Autodesk Inventor part; units mm, degrees
ref_plane "YZ Plane" through (0, 0, 0) normal (1, 0, 0) x (0, 1, 0)
ref_plane "XZ Plane" through (0, 0, 0) normal (0, 1, 0) x (-1, 0, 0)
ref_plane "XY Plane" through (0, 0, 0) normal (0, 0, 1) x (1, 0, 0)
sketch "Sketch1" plane through (0, 0, 0) normal (0, 0, 1) x (1, 0, 0)
  line L0 (0, 0) -> (310, 0)
  line L1 (310, 0) -> (310, 40)
  line L2 (310, 40) -> (0, 40)
  line L3 (0, 40) -> (0, 0)
  dimension "d1" = 40
  dimension "d2" = 310
extrude "Plate1" add sketch "Sketch1" along normal blind 2
sketch "Sketch2" plane through (310, 38, 2) normal (0, 1, 0) x (-1, 0, 0)
  line L0 (310, 0) -> (0, 0)
  line L1 (0, 0) -> (0, -25)
  line L2 (0, -25) -> (310, -25)
  line L3 (310, -25) -> (310, 0)
edge flange "Flange1" height 25 angle 90 thickness 2 bend radius 2 thickness toward (0, 1, 0) relief tear relief width 2 relief depth 1 edges at (155, 40, 0) wall of the first edge with corners at (0, 38, 2) (310, 38, 2) (310, 38, -23) (0, 38, -23)
bend "Bend1"
corner "Corner1"
sketch "Sketch3" plane through (0, 2, 2) normal (0, -1, 0) x (1, 0, 0)
  line L0 (310, 0) -> (0, 0)
  line L1 (0, 0) -> (0, -12)
  line L2 (0, -12) -> (310, -12)
  line L3 (310, -12) -> (310, 0)
edge flange "Flange2" height 12 angle 90 thickness 2 bend radius 2 thickness toward (0, -1, 0) relief tear relief width 2 relief depth 1 edges at (155, 0, 0) wall of the first edge with corners at (310, 2, 2) (0, 2, 2) (0, 2, -10) (310, 2, -10)
bend "Bend2"
corner "Corner2"
sketch "Sketch4" plane through (0, 0, 2) normal (0, 0, 1) x (1, 0, 0)
  arc A0 (146.75, 13.9172) -> (163.25, 13.9172) centre (155, 20) ccw
  line L0 (0, 4) -> (0, 36)
  line L1 (0, 40) -> (310, 40)
  line L2 (146.75, 26.0828) -> (146.75, 13.9172)
  line L3 (163.25, 26.0828) -> (163.25, 13.9172)
  arc A1 (146.75, 26.0828) -> (146.75, 13.9172) centre (155, 20) ccw construction
  arc A2 (163.25, 26.0828) -> (146.75, 26.0828) centre (155, 20) ccw
  arc A3 (163.25, 13.9172) -> (163.25, 26.0828) centre (155, 20) ccw construction
  point P0 (0, 0)
  point P1 (0, 20)
  point P2 (155, 40)
  dimension "d25" = 20.5
  dimension "d26" = 16.5
extrude "Cut1" cut sketch "Sketch4" against normal blind 2
sketch "Sketch5" plane through (0, 0, 2) normal (0, 0, 1) x (1, 0, 0)
  line L0 (310, 4) -> (0, 4)
  line L1 (145, 4) -> (165, 4)
  line L2 (165, 4) -> (165, -2)
  line L3 (165, -2) -> (145, -2)
  line L4 (145, -2) -> (145, 4)
  point P0 (0, 0)
  point P1 (155, -2)
  point P2 (155, 4)
  dimension "d27" = 20
  dimension "d28" = 6
extrude "Cut2" cut sketch "Sketch5" against normal through all
equation "\"d23\" = Thickness"
equation "\"d29\" = Thickness"
equation "\"d3\" = BendReliefWidth"
equation "\"d4\" = BendReliefDepth"
equation "\"d5\" = MinimumRemnant"
equation "\"d6\" = BendRadius"
equation "\"d9\" = BendRadius"
equation "\"d10\" = CornerReliefSize"
equation "\"d11\" = GapSize"
equation "\"d12\" = JacobiRadiusSize"
equation "\"d13\" = BendReliefWidth"
equation "\"d14\" = BendReliefDepth"
equation "\"d15\" = MinimumRemnant"
equation "\"d16\" = BendRadius"
equation "\"d19\" = BendRadius"
equation "\"d20\" = CornerReliefSize"
equation "\"d21\" = GapSize"
equation "\"d22\" = JacobiRadiusSize"
equation "\"BendRadius\" = Thickness"
equation "\"BendReliefWidth\" = Thickness"
equation "\"BendReliefDepth\" = 0.5 * Thickness"
equation "\"CornerReliefSize\" = 4 * Thickness"
equation "\"MinimumRemnant\" = 2 * Thickness"
equation "\"TransitionRadius\" = BendRadius"
equation "\"JacobiRadiusSize\" = BendRadius"
equation "\"GapSize\" = Thickness"
equation "\"d0\" = BendRadius"
Model file for the job. Use its own axes, mm. A direction names the side the tool comes from. Coordinates: 2 decimals unless noted, no trailing zeros. Loops run counter-clockwise (first coordinate to the right, second up) from the corner with the lowest first, then second, coordinate; pieces in that order, holes last. Notation, with made-up numbers: M 2.5,34.5 L 30.5,34.5 A26 ccw 30.5,53.5 Z; hole C 23.5,30.25 d7. An arc over 180 degrees is marked long. Use CSV: the item, a comma, the result in double quotes. Start each with the question number.
1. Probe probe 1 along Y at (x, z) = (48, -8); probe 2 along Y at (x, z) = (152.5, -6.5); probe 3 along Z at (x, y) = (163, 33). List the from-to ranges inside material, lowest first. Write a range as [from, to].
2. Band-saw the part on B-B, the plane y = 17.5. List the corners of the cut face in (x, z), then the cut area to 3 significant figures.
3. Two-plate mould, pull along Y, no slides. Class faces 1 (the flat face through (236, 0, -6)), 2 (the flat face through (236, 2, -6)), 3 (the flat face through (157, 40, -13)), 4 (the flat face through (310, 23, 1)): pulls with the +Y half, pulls with the -Y half, needs draft (parallel to the pull), parting line crosses it, or undercut.
4. Band-saw the part on C-C, the plane x = 105. List the corners of the cut face in (y, z), then the cut area to 3 significant figures.
5. Flat gauge pins, fed straight in: pin 1 (10 mm diameter, centred on y = 31.5, z = -11, fed in from -X); pin 2 (2 mm diameter, centred on y = 1, z = -2.5, fed in from -X); pin 3 (6.5 mm diameter, centred on x = 203, z = -14, fed in from -Y); pin 4 (2 mm diameter, centred on x = 92.5, y = 0.5, fed in from -Z). Where does each tip first touch, or does it go through?
6. Band-saw the part on A-A, the plane z = -6.75. List the corners of the cut face in (x, y), then the cut area to 3 significant figures.
7. Tool access for faces 5 (the flat face through (153, 31, 2)), 6 (the flat face through (71, 2, -6)): list every direction of +Z, -Z, +X, -X, +Y, -Y with a clear straight run to the whole face (end or side of a thin tool).
Entries:
1,probe 1,"y = [0, 2], [38, 40]"
1,probe 2,"y = [38, 40]"
1,probe 3,"z = [0, 2]"
2,outline,"M 0,0 L 146.75,0 L 146.75,2 L 0,2 Z; M 163.25,0 L 310,0 L 310,2 L 163.25,2 Z"
2,area,"587 mm2"
3,face 1,"pulls with the -Y half"
3,face 2,"undercut"
3,face 3,"pulls with the +Y half"
3,face 4,"needs draft"
4,outline,"M 0,-10 L 2,-10 L 2,-2 A2 cw 4,0 L 36,0 A2 cw 38,-2 L 38,-23 L 40,-23 L 40,-2 A4 ccw 36,2 L 4,2 A4 ccw 0,-2 Z"
4,area,"141 mm2"
5,pin 1,"passes through"
5,pin 2,"stops at x = 0"
5,pin 3,"stops at y = 38"
5,pin 4,"stops at z = -10"
6,outline,"M 0,0 L 145,0 L 145,2 L 0,2 Z; M 0,38 L 310,38 L 310,40 L 0,40 Z; M 165,0 L 310,0 L 310,2 L 165,2 Z"
6,area,"1,200 mm2"
7,face 5,"+Z, +X, -X, +Y, -Y"
7,face 6,"-Z, +X, -X"
